from build123d import *

# Parameters (mm, degrees)
F0_W     = 55.88
F0_H     = 76.2
F1_DEPTH = 12.7
F2_W     = 53.34
F2_H     = 73.66
F3_DEPTH = 10.16
F4_W     = 12.7
F4_H     = 25.4
F5_DEPTH = 6.35
F6_W     = 12.7
F6_H     = 25.4
F7_DEPTH = 6.35
F8_W     = 3.937
F8_H     = 22.86
F9_DEPTH = 25.4


with BuildPart() as f1:
    # F0 (on Front) → F1 (new body)
    with BuildSketch(Plane.XZ):
        Rectangle(F0_W, F0_H)
    extrude(amount=F1_DEPTH)

    # F2 (on face) → F3 (cut)
    with BuildSketch(Plane.XZ.offset(12.7)):
        Rectangle(F2_W, F2_H)
    extrude(amount=-F3_DEPTH, mode=Mode.SUBTRACT)

    # F4 (on face) → F5 (join)
    with BuildSketch(Plane.YZ.offset(27.94)):
        with Locations((-6.35, 0)):
            Rectangle(F4_W, F4_H)
    extrude(amount=F5_DEPTH)

    # F6 (on face) → F7 (join)
    with BuildSketch(Plane(origin=(-27.94, 0, 0), x_dir=(0, -1, 0), z_dir=(-1, 0, 0))):
        with Locations((6.35, 0)):
            Rectangle(F6_W, F6_H)
    extrude(amount=F7_DEPTH)

    # F8 (on face) → F9 (cut)
    with BuildSketch(Plane.XZ.offset(12.7)):
        with Locations((-31.115, 0)):
            Rectangle(F8_W, F8_H)
        with Locations((31.115, 0)):
            Rectangle(F8_W, F8_H)
    extrude(amount=-F9_DEPTH, mode=Mode.SUBTRACT)


solid = f1.part
Geometry: final body of the model. Coordinates: model frame, mm. A direction names the side the tool comes from. Coordinates: 2 decimals unless noted, no trailing zeros. Order: outer loops, then holes, each group sorted by start corner. A loop starts at its lowest first (then second) coordinate and runs counter-clockwise, first axis right, second up.
(1) Section query D-D (z = -16.5). Return the cut outline in (x, y).
(2) Section query B-B (y = -8). Return the cut outline in (x, z).
(3) Access query for faces 1 (the face through (27.94, -6, 25)), 2 (the face through (-27.94, -6, -26)), 3 (the face through (0, -8, 36.83)). Directions: +Z, -Z, +X, -X, +Y, -Y. A direction counts if a zero-diameter tool reaches every point of the face in a straight line with its end or side. Return the directions, or none.
(4) First-contact query: pin 1 (4 mm diameter, centred on y = -4, z = -21, fed in from -X); pin 2 (3 mm diameter, centred on y = -5, z = -21, fed in from +X); pin 3 (3 mm diameter, centred on x = 31.5, y = -9, fed in from +Z). Flat tips, straight axial feed; report the tip coordinate or a pass-through.
(5) Section query C-C (y = -1.25). Return the cut outline in (x, z).
(6) Section query A-A (z = 6.5). Return the cut outline in (x, y), plus the area to 3 significant figures.
(7) Material intervals for probe 1 along X at (y, z) = (-11, -5.5); probe 2 along Z at (x, y) = (21.5, -9.5); probe 3 along X at (y, z) = (-12, -27), sorted ascending.
Solution:
1. outline: (-27.94, -12.7) - (-26.67, -12.7) - (-26.67, -2.54) - (26.67, -2.54) - (26.67, -12.7) - (27.94, -12.7) - (27.94, 0) - (-27.94, 0) - close
2. outline: (-34.29, -12.7) - (-27.94, -12.7) - (-27.94, -38.1) - (27.94, -38.1) - (27.94, -12.7) - (34.29, -12.7) - (34.29, 12.7) - (27.94, 12.7) - (27.94, 38.1) - (-27.94, 38.1) - (-27.94, 12.7) - (-34.29, 12.7) - close; hole (-33.08, -11.43) - (-29.15, -11.43) - (-29.15, 11.43) - (-33.08, 11.43) - close; hole (-26.67, -36.83) - (26.67, -36.83) - (26.67, 36.83) - (-26.67, 36.83) - close; hole (29.15, -11.43) - (33.08, -11.43) - (33.08, 11.43) - (29.15, 11.43) - close
3. face 1: +Z, +X, +Y, -Y
3. face 2: -Z, -X, +Y, -Y
3. face 3: -Y
4. pin 1: stops at x = -27.94
4. pin 2: stops at x = 27.94
4. pin 3: stops at z = 12.7
5. outline: (-34.29, -12.7) - (-27.94, -12.7) - (-27.94, -38.1) - (27.94, -38.1) - (27.94, -12.7) - (34.29, -12.7) - (34.29, 12.7) - (27.94, 12.7) - (27.94, 38.1) - (-27.94, 38.1) - (-27.94, 12.7) - (-34.29, 12.7) - close; hole (-33.08, -11.43) - (-29.15, -11.43) - (-29.15, 11.43) - (-33.08, 11.43) - close; hole (29.15, -11.43) - (33.08, -11.43) - (33.08, 11.43) - (29.15, 11.43) - close
6. outline: (-34.29, -12.7) - (-33.08, -12.7) - (-33.08, 0) - (-34.29, 0) - close; (-29.15, -12.7) - (-26.67, -12.7) - (-26.67, -2.54) - (26.67, -2.54) - (26.67, -12.7) - (29.15, -12.7) - (29.15, 0) - (-29.15, 0) - close; (33.08, -12.7) - (34.29, -12.7) - (34.29, 0) - (33.08, 0) - close
6. area: 229 mm2
7. probe 1: x = -34.29 to -33.08, -29.15 to -26.67, 26.67 to 29.15, 33.08 to 34.29
7. probe 2: z = -38.1 to -36.83, 36.83 to 38.1
7. probe 3: x = -27.94 to -26.67, 26.67 to 27.94
